```python
from build123d import *

# Parameters (mm, degrees)
SKETCH1_R           = 2
SKETCH1_W           = 6.5
SKETCH1_H           = 19
SKETCH1_W_2         = 45
SKETCH1_H_2         = 15
BOSS_EXTRUDE1_DEPTH = 3
FILLET1_R           = 3
FILLET2_R           = 2


with BuildPart() as part:
    # Sketch1 → Boss-Extrude1 (new body)
    with BuildSketch(Plane(origin=(0, 0, 0), x_dir=(1, 0, 0), z_dir=(0, 1, 0))):
        with BuildLine():
            Line((-22.5, 2), (-22.5, -17))
            Line((-22.5, -17), (22.5, -17))
            Line((22.5, -17), (22.5, -6.936491673))
            ThreePointArc((22.5, -6.936491673), (21, -5), (22.5, -3.063508327))
            Line((22.5, -3.063508327), (22.5, 2))
            Line((22.5, 2), (-22.5, 2))
        make_face()
        with Locations((-15, -12)):
            Circle(SKETCH1_R, mode=Mode.SUBTRACT)
        with Locations((15, -12)):
            Circle(SKETCH1_R, mode=Mode.SUBTRACT)
        with Locations((-25.75, -7.5)):
            Rectangle(SKETCH1_W, SKETCH1_H)
        with Locations((-25, -5)):
            Circle(SKETCH1_R, mode=Mode.SUBTRACT)
        with Locations((0, 9.5)):
            Rectangle(SKETCH1_W_2, SKETCH1_H_2)
        with Locations((-15, 12)):
            Circle(SKETCH1_R, mode=Mode.SUBTRACT)
        with Locations((15, 12)):
            Circle(SKETCH1_R, mode=Mode.SUBTRACT)
        with BuildLine():
            Line((22.5, -6.936491673), (22.5, -17))
            Line((22.5, -17), (31, -17))
            Line((31, -17), (31, 2))
            Line((31, 2), (22.5, 2))
            Line((22.5, 2), (22.5, -3.063508327))
            ThreePointArc((22.5, -3.063508327), (22.747991415, -3.015940607), (23, -3))
            Line((23, -3), (26, -3))
            ThreePointArc((26, -3), (28, -5), (26, -7))
            Line((26, -7), (23, -7))
            ThreePointArc((23, -7), (22.747991415, -6.984059393), (22.5, -6.936491673))
        make_face()
    extrude(amount=BOSS_EXTRUDE1_DEPTH)

    # Fillet1
    fillet1_edges = [part.edges().sort_by_distance(p)[0] for p in [
        (31, 1.5, -2),
        (31, 1.5, 17),
        (-29, 1.5, 17),
        (-29, 1.5, -2),
        (-22.5, 1.5, -17),
        (22.5, 1.5, -17),
    ]]
    fillet(fillet1_edges, radius=FILLET1_R)

    # Fillet2
    fillet2_edges = [part.edges().sort_by_distance(p)[0] for p in [
        (-22.5, 1.5, -2),
        (22.5, 1.5, -2),
    ]]
    fillet(fillet2_edges, radius=FILLET2_R)


solid = part.part
```
Read the model definition and answer for the solid it produces. Units are mm, in the model's axes. A direction names the side the tool comes from. Give positions to 0.01 mm unless a question says otherwise; leave off trailing zeros. Order: outer loops, then holes, each group sorted by start corner. A loop starts at its lowest first (then second) coordinate and runs counter-clockwise, first axis right, second up.
(1) Given pin 1 (3 mm diameter, centred on x = -15, z = -12, fed in from -Y); pin 2 (1.5 mm diameter, centred on y = 1.5, z = -7.5, fed in from -X); pin 3 (1.5 mm diameter, centred on y = 1, z = -6.5, fed in from +X); pin 4 (0.8 mm diameter, centred on x = -25.5, y = 1, fed in from -Z), each flat-ended and moving along its own axis, determine where each tip first touches the part or whether it passes through.
(2) Find section A-A (z = 5). Give the vertices of the cut face in (x, y).
(3) For a pull along X with two mould halves and no side action, classify faces 1 (the flat face through (-29, 1, 8)), 2 (the flat face through (-25, 1, -2)), 3 (the cylindrical face through (-15, 1, -14)) as released by +X, released by -X, zero draft, split by the parting line, or undercut.
(4) Find section C-C (y = 1). Give the vertices of the cut face in (x, z), plus the area to 3 significant figures.
(5) Straight lines are drawn through the part: L1, parallel to X at y = 1.35, z = 12; L2, parallel to X at y = 0.1, z = -12; L3, parallel to Z at x = 15, y = 2.3. For each, find the intervals that lie inside material, in ascending order.
(6) Find section D-D (z = -1). Give the vertices of the cut face in (x, y), plus the area to 3 significant figures.
(7) Find section B-B (x = 15). Give the vertices of the cut face in (y, z), plus the area to 3 significant figures.
(8) For faces 4 (the flat face through (31, 1, 8)), 5 (the flat face through (24, 1, 3)), 6 (the flat face through (26, 1, -2)), 7 (the flat face through (1, 0, 0)), 8 (the flat face through (-22.5, 1, -9)), determine the directions among +Z, -Z, +X, -X, +Y, -Y from which every point of the face is accessible in a straight line to the end or side of a thin tool.
Result sheet:
1. pin 1: passes through
1. pin 2: stops at x = -22.5
1. pin 3: stops at x = 22.5
1. pin 4: stops at z = -2
2. outline: (-29, 0) - (-27, 0) - (-27, 3) - (-29, 3) - close; (-23, 0) - (21, 0) - (21, 3) - (-23, 3) - close; (28, 0) - (31, 0) - (31, 3) - (28, 3) - close
3. face 1: released by -X
3. face 2: zero draft
3. face 3: undercut
4. outline: (-29, 1) arc R3 ccw to (-26, -2) - (-24.5, -2) arc R2 cw to (-22.5, -4) - (-22.5, -14) arc R3 ccw to (-19.5, -17) - (19.5, -17) arc R3 ccw to (22.5, -14) - (22.5, -4) arc R2 cw to (24.5, -2) - (28, -2) arc R3 ccw to (31, 1) - (31, 14) arc R3 ccw to (28, 17) - (-26, 17) arc R3 ccw to (-29, 14) - close; hole circle Ø4 at (-25, 5); hole circle Ø4 at (-15, -12); hole circle Ø4 at (-15, 12); hole circle Ø4 at (15, -12); hole circle Ø4 at (15, 12); hole (23, 3) - (26, 3) arc R2 ccw to (26, 7) - (23, 7) arc R2 ccw to start
4. area: 1,720 mm2
5. L1: x = -29 to -17, -13 to 13, 17 to 31
5. L2: x = -22.5 to -17, -13 to 13, 17 to 22.5
5. L3: z = -17 to -14, -10 to 10, 14 to 17
6. outline: (-28.24, 0) - (30.24, 0) - (30.24, 3) - (-28.24, 3) - close
6. area: 175 mm2
7. outline: (0, -17) - (3, -17) - (3, -14) - (0, -14) - close; (0, -10) - (3, -10) - (3, 10) - (0, 10) - close; (0, 14) - (3, 14) - (3, 17) - (0, 17) - close
7. area: 78.0 mm2
8. face 4: +Z, -Z, +X, +Y, -Y
8. face 5: +Y, -Y
8. face 6: -Z, +X, +Y, -Y
8. face 7: +Z, -Z, +X, -X, -Y
8. face 8: -Z, -X, +Y, -Y
